from build123d import *

# Parameters (mm, degrees)
BOSS_EXTRUDE1_DEPTH          = 2.4
SKETCH2_W                    = 15.6
SKETCH2_H                    = 2.4
BOSS_EXTRUDE2_DEPTH          = 6.32
BOSS_EXTRUDE3_DEPTH          = 2.4
BOSS_EXTRUDE4_DEPTH          = 2.4
F_6_0_6_DIAMETER_HOLE1_D     = 6
F_6_0_6_DIAMETER_HOLE1_DEPTH = 18.00005
F_6_0_6_DIAMETER_HOLE2_D     = 6
F_6_0_6_DIAMETER_HOLE2_DEPTH = 18.00005
F_6_0_6_DIAMETER_HOLE3_D     = 6
F_6_0_6_DIAMETER_HOLE3_DEPTH = 18.00005


with BuildPart() as part:
    # Boss-Extrude1: read off the stored shape, not the designer's step
    # Boss-Extrude1 outline → Boss-Extrude1 (new body)
    with BuildSketch(Plane(origin=(0, 0, 0), x_dir=(1, 0, 0), z_dir=(0, 1, 0))):
        Polygon((2.4, -18), (8.72, -18), (18, -8.72), (2.4, -8.72), align=None)
    extrude(amount=BOSS_EXTRUDE1_DEPTH)

    # Sketch2 → Boss-Extrude2 (add)
    with BuildSketch(Plane(origin=(0, 0, 8.72), x_dir=(-1, 0, 0), z_dir=(0, 0, -1))):
        with Locations((-10.2, 1.2)):
            Rectangle(SKETCH2_W, SKETCH2_H)
    extrude(amount=BOSS_EXTRUDE2_DEPTH)

    # Sketch3 → Boss-Extrude3 (add)
    with BuildSketch(Plane(origin=(0, 0, 2.4), x_dir=(-1, 0, 0), z_dir=(0, 0, -1))):
        Polygon((-2.4, 0), (-18, 0), (-18, 8.72), (-8.72, 18), (-2.4, 18), align=None)
    extrude(amount=BOSS_EXTRUDE3_DEPTH)

    # Sketch4 → Boss-Extrude4 (add)
    with BuildSketch(Plane.ZY.offset(-2.4)):
        Polygon((0, 18), (8.72, 18), (18, 8.72), (18, 0), (0, 0), align=None)
    extrude(amount=BOSS_EXTRUDE4_DEPTH)

    # Ø6.0 (6) Diameter Hole1
    with Locations(Plane.ZY):
        with Locations((9.9, 9.9)):
            Hole(F_6_0_6_DIAMETER_HOLE1_D / 2, depth=F_6_0_6_DIAMETER_HOLE1_DEPTH)

    # Ø6.0 (6) Diameter Hole2
    with Locations(Plane(origin=(0, 0, 0), x_dir=(-1, 0, 0), z_dir=(0, 0, -1))):
        with Locations((-9.9, 9.9)):
            Hole(F_6_0_6_DIAMETER_HOLE2_D / 2, depth=F_6_0_6_DIAMETER_HOLE2_DEPTH)

    # Ø6.0 (6) Diameter Hole3
    with Locations(Plane(origin=(0, 0, 0), x_dir=(-1, 0, 0), z_dir=(0, -1, 0))):
        with Locations((-9.9, -9.9)):
            Hole(F_6_0_6_DIAMETER_HOLE3_D / 2, depth=F_6_0_6_DIAMETER_HOLE3_DEPTH)


solid = part.part
The model under review builds one solid part; all positions refer to its coordinate system, in mm. A direction names the side the tool comes from. Round coordinates to 2 decimals unless told otherwise and drop trailing zeros. Order: outer loops, then holes, each group sorted by start corner. A loop starts at its lowest first (then second) coordinate and runs counter-clockwise, first axis right, second up. Notation, with made-up numbers: (25, 0.25) -> (52, 0.25) arc R17 cw to (52, 13.25) -> close; hole circle Ø3 at (-40, 84.25). An arc over 180 degrees is marked (long way). Write item = value, one per line. Start each with the question number.
Item 1: For line 1 along Y through (x, z) = (7.5, 13.5), list the stretches that pass through material, from the lowest coordinate up.
Item 2: Consider section C-C on y = 3. Write out the cut boundary in (x, z).
Item 3: Mouldability with a two-part tool opening along Y and no side actions: class faces 1 (the face through (9.25, 6.97, 1.22)), 2 (the face through (1.22, 13.42, 13.3)), 3 (the face through (0, 7, 7)), 4 (the face through (1.2, 8.1, 12.3)) as released by +Y, released by -Y, zero draft, split by the parting line, or undercut.
Item 4: Clearance check with flat-ended pins moving along their axes: pin 1 Ø9.5 at (y, z) = (9.9, 9.9) entering from +X; pin 2 Ø2 at (x, z) = (3.5, 8.5) entering from -Y; pin 3 Ø4.5 at (x, z) = (11, 12.5) entering from +Y. State where each tip first meets the part, or that it passes through.
Item 5: For faces 5 (the face through (8, 7, 2.4)), 6 (the face through (18, 2, 3)), list the 3-axis set-ups (+Z, -Z, +X, -X, +Y, -Y) from which the entire face can be reached by the end or side of a thin tool; tool diameter is ignored.
Item 6: Consider section D-D on x = 2. Write out the cut boundary in (y, z), plus the area to 3 significant figures.
Item 7: Consider section A-A on x = 9.9. Write out the cut boundary in (y, z).
Conclusion:
q1.line_1 = 0 to 2.4
q2.outline = (0, 0) -> (18, 0) -> (18, 2.4) -> (2.4, 2.4) -> (2.4, 18) -> (0, 18) -> close
q3.face_1 = undercut
q3.face_2 = released by +Y
q3.face_3 = zero draft
q3.face_4 = undercut
q4.pin_1 = 2.4
q4.pin_2 = 0
q4.pin_3 = 2.4
q5.face_5 = +Z, +X, +Y
q5.face_6 = +Z, -Z, +X, +Y, -Y
q6.outline = (0, 0) -> (18, 0) -> (18, 8.72) -> (8.72, 18) -> (0, 18) -> close; hole circle Ø6 at (9.9, 9.9)
q6.area = 253 mm2
q7.outline = (0, 0) -> (6.9, 0) -> (6.9, 2.4) -> (2.4, 2.4) -> (2.4, 6.9) -> (0, 6.9) -> close; (0, 12.9) -> (2.4, 12.9) -> (2.4, 16.82) -> (0, 16.82) -> close; (12.9, 0) -> (16.82, 0) -> (16.82, 2.4) -> (12.9, 2.4) -> close
